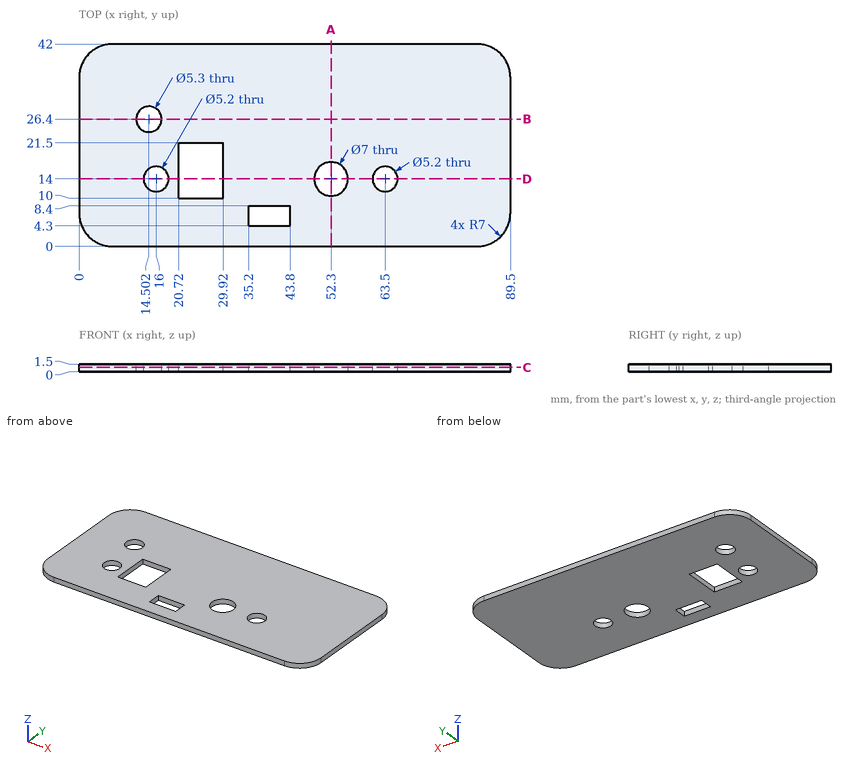
Check sheet for the drawn part. Datum: minimum x, y, z corner. Units: mm. Give positions to 0.01 mm unless a question says otherwise; leave off trailing zeros. Loops run counter-clockwise (first coordinate to the right, second up) from the corner with the lowest first, then second, coordinate; pieces in that order, holes last. Notation, with made-up numbers: M -38.75,74.25 L -27.75,74.25 A35 cw -27.75,106.25 Z; hole C 29,83 d7. An arc over 180 degrees is marked long. Return JSON: item names as keys, results as strings.
1) Material ranges on L1, parallel to Y at x = 16, z = 0.55 (1 decimal); L2, parallel to Y at x = 28, z = 1.35; L3, parallel to Y at x = 52.3, z = 0.45, recorded low to high. Write a range as [from, to].
Findings:
{"L1": "y = [0, 11.4], [16.6, 24.2], [28.6, 42]", "L2": "y = [0, 10], [21.5, 42]", "L3": "y = [0, 10.5], [17.5, 42]"}
2) Section check B-B, the plane y = 26.4. Enter the section's corners in (x, z), and give its area (3 significant figures).
Findings:
{"outline": "M 0,0 L 11.85,0 L 11.85,1.5 L 0,1.5 Z; M 17.15,0 L 89.5,0 L 89.5,1.5 L 17.15,1.5 Z", "area": "126 mm2"}
3) Section check A-A, the plane x = 52.3. Enter the section's corners in (y, z), and give its area (3 significant figures).
Findings:
{"outline": "M 0,0 L 10.5,0 L 10.5,1.5 L 0,1.5 Z; M 17.5,0 L 42,0 L 42,1.5 L 17.5,1.5 Z", "area": "52.5 mm2"}
4) Section check D-D, the plane y = 14. Enter the section's corners in (x, z).
Findings:
{"outline": "M 0,0 L 13.4,0 L 13.4,1.5 L 0,1.5 Z; M 18.6,0 L 20.72,0 L 20.72,1.5 L 18.6,1.5 Z; M 29.92,0 L 48.8,0 L 48.8,1.5 L 29.92,1.5 Z; M 55.8,0 L 60.9,0 L 60.9,1.5 L 55.8,1.5 Z; M 66.1,0 L 89.5,0 L 89.5,1.5 L 66.1,1.5 Z"}
5) Section check C-C, the plane z = 0.9. Enter the section's corners in (x, y).
Findings:
{"outline": "M 0,7 A7 ccw 7,0 L 82.5,0 A7 ccw 89.5,7 L 89.5,35 A7 ccw 82.5,42 L 7,42 A7 ccw 0,35 Z; hole C 14.5,26.4 d5.3; hole C 16,14 d5.2; hole M 20.72,10 L 29.92,10 L 29.92,21.5 L 20.72,21.5 Z; hole M 35.2,4.3 L 43.8,4.3 L 43.8,8.4 L 35.2,8.4 Z; hole C 52.3,14 d7; hole C 63.5,14 d5.2"}
